Verification items for the finished model (mm, model axes). Face numbers are marked on the shaded views. A direction names the side the tool comes from. Round coordinates to 2 decimals unless told otherwise and drop trailing zeros. Loops run counter-clockwise (first coordinate to the right, second up) from the corner with the lowest first, then second, coordinate; pieces in that order, holes last. Notation, with made-up numbers: (64, 13.25) -> (107, 13.25) arc R26 ccw to (107, 38.25) -> close; hole circle Ø2 at (23, 31.25). An arc over 180 degrees is marked (long way). Write item = value, one per line.
```python
from build123d import *

# Parameters (mm, degrees)
F0_W      = 100
F0_H      = 80
F1_DEPTH  = 45
F2_R      = 7.5
F3_DEPTH  = 30
F4_R      = 70
F5_DEPTH  = 20
F6_W      = 20
F6_H      = 15
F7_DEPTH  = 10
F9_DEPTH  = 25.001
F11_DEPTH = 80.001


with BuildPart() as f1:
    # F0 (on Top) → F1 (new body)
    with BuildSketch(Plane.XY):
        with Locations((50, 40)):
            Rectangle(F0_W, F0_H)
    extrude(amount=F1_DEPTH)

    # F2 (on face) → F3 (cut)
    with BuildSketch(Plane.XY.offset(45)):
        with Locations((60, 52.916668)):
            Circle(F2_R)
    extrude(amount=-F3_DEPTH, mode=Mode.SUBTRACT)

    # F4 (on face) → F5 (cut)
    with BuildSketch(Plane.XY.offset(45)):
        Circle(F4_R)
    extrude(amount=-F5_DEPTH, mode=Mode.SUBTRACT)

    # F6 (on face) → F7 (join)
    with BuildSketch(Plane.XY.offset(25)):
        with Locations((10, 7.5)):
            Rectangle(F6_W, F6_H)
    extrude(amount=F7_DEPTH)

    # F8 (on face) → F9 (cut, through all)
    with BuildSketch(Plane.XY.offset(25)):
        with BuildLine():
            ThreePointArc((63.245553, 30), (51.453576, 47.460821), (35, 60.621778))
            Line((35, 60.621778), (35, 30))
            Line((35, 30), (63.245553, 30))
        make_face()
    extrude(amount=-F9_DEPTH, mode=Mode.SUBTRACT)

    # F10 (on face) → F11 (cut, through all)
    with BuildSketch(Plane.XZ):
        with BuildLine():
            ThreePointArc((74.583337, 45), (91.596706, 24.931549), (100, 0))
            Line((100, 0), (100, 45))
            Line((100, 45), (74.583337, 45))
        make_face()
    extrude(amount=-F11_DEPTH, mode=Mode.SUBTRACT)


solid = f1.part
```
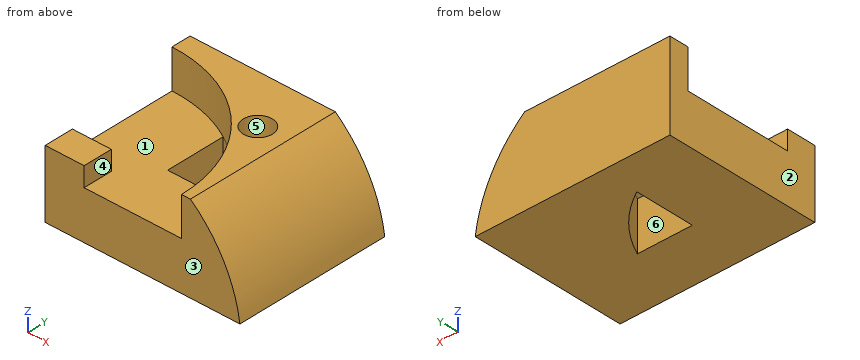
(1) Sectioned sample at B-B, the plane x = 60. Record the cut outline in (y, z).
Filled sheet:
outline = (0, 0) -> (30, 0) -> (30, 25) -> (0, 25) -> close; (36.06, 0) -> (80, 0) -> (80, 45) -> (60.42, 45) -> (60.42, 15) -> (45.42, 15) -> (45.42, 45) -> (36.06, 45) -> close
(2) Sectioned sample at A-A, the plane z = 31. Record the cut outline in (x, y), and give its area (3 significant figures).
Filled sheet:
outline = (0, 0) -> (20, 0) -> (20, 15) -> (0, 15) -> close; (0, 70) arc R70 cw to (70, 0) -> (87.75, 0) -> (87.75, 80) -> (0, 80) -> close; hole circle Ø15 at (60, 52.92)
area = 3,290 mm2
(3) Set-up check for the marked faces 4, 5 and 6: record each of +Z, -Z, +X, -X, +Y, -Y from which the full face is reachable in a straight line by a thin tool's end or side.
Filled sheet:
face_4 = +Z, -Y
face_5 = +Z
face_6 = +Z, -Z
(4) Sectioned sample at C-C, the plane y = 75.5. Record the cut outline in (x, z).
Filled sheet:
outline = (0, 0) -> (100, 0) arc R70 ccw to (74.58, 45) -> (0, 45) -> close
(5) Go/stop test with flat-tipped pins: pin 1 Ø1 at (x, y) = (48, 48.5) entering from +Z; pin 2 Ø6 at (y, z) = (27, 14.5) entering from +X; pin 3 Ø16.5 at (x, y) = (6, 8) entering from +Z; pin 4 Ø2 at (y, z) = (21.5, 34) entering from +X. Record where each tip stops, or that it passes through.
Filled sheet:
pin_1 = through
pin_2 = 97.42
pin_3 = 35
pin_4 = 86.27
(6) Draft check along X on the marked faces 1, 2 and 3. Enter one of: released by +X, released by -X, zero draft, split by the parting line, or undercut.
Filled sheet:
face_1 = undercut
face_2 = released by -X
face_3 = zero draft
(7) Sectioned sample at D-D, the plane z = 22. Record the cut outline in (x, y), and give its area (3 significant figures).
Filled sheet:
outline = (0, 0) -> (93.16, 0) -> (93.16, 80) -> (0, 80) -> close; hole (35, 30) -> (63.25, 30) arc R70 ccw to (35, 60.62) -> close; hole circle Ø15 at (60, 52.92)
area = 6,760 mm2
(8) Material ranges on probe 1 along X at (y, z) = (50.5, 28); probe 2 along Z at (x, y) = (15.5, 35.5); probe 3 along X at (y, z) = (47.5, 14.5), recorded low to high. Write a range as from..to.
Filled sheet:
probe_1 = 48.47..52.9, 67.1..89.76
probe_2 = 0..25
probe_3 = 0..35, 51.42..96.41
